Input: dimensioned drawing with shaded views. Units: mm. Origin: part minimum x, y, z. A direction names the side the tool comes from. Give positions to 0.01 mm unless a question says otherwise; leave off trailing zeros. Write each loop counter-clockwise with the first axis right and the second up, starting at its lowest first coordinate (ties: lowest second). Pieces come first, ordered by that corner, then holes.
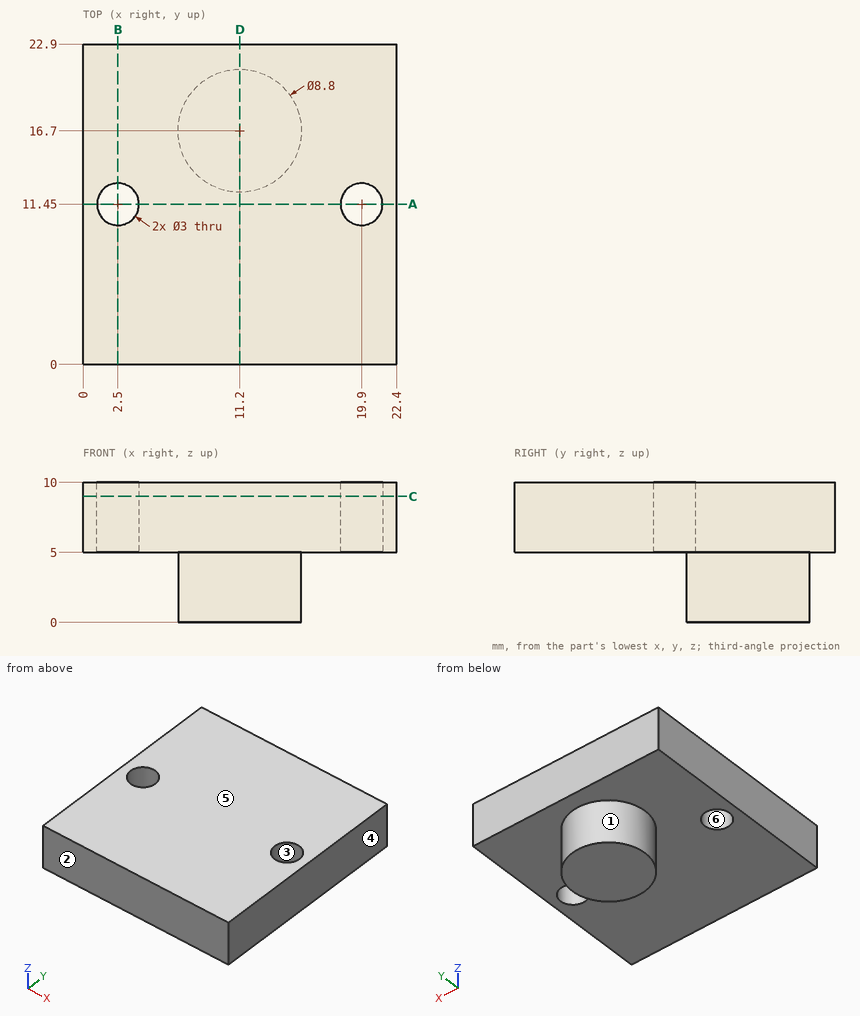
Item 1: Section C-C (z = 9). Return loops of the section in (x, y).
Item 2: Ray query, line 1 (Y direction, x = 19.9, z = 6.7); line 2 (Z direction, x = 1.75, y = 4.25); line 3 (Y direction, x = 11.5, z = 2.25). Return the intervals inside material, ascending.
Item 3: Set-up query: the marked faces 1 and 2. Return all of +Z, -Z, +X, -X, +Y, -Y with unobstructed straight access to the full face (end or side cutting, diameter ignored); none if empty.
Item 4: Section D-D (x = 11.2). Return loops of the section in (y, z).
Item 5: Mould query, pull axis X, two halves, no side actions, for the marked faces 3, 4, 5 and 6. Classes: +X half, -X half, draft (parallel to the pull), parting line (faces both ways), or undercut.
Item 6: Section B-B (x = 2.5). Return loops of the section in (y, z), and give its area (3 significant figures).
Item 7: Section A-A (y = 11.45). Return loops of the section in (x, z), and give its area (3 significant figures).
Item 8: Pin query (flat end, axial travel): pin 1 (1 mm diameter, centred on y = 15.5, z = 4, fed in from -X); pin 2 (5 mm diameter, centred on x = 19.9, y = 11.45, fed in from -Z). Return the tip coordinate at first contact, or that it passes through.
Solved:
1. outline: (0, 0) - (22.4, 0) - (22.4, 22.9) - (0, 22.9) - close; hole circle Ø3 at (2.5, 11.45); hole circle Ø3 at (19.9, 11.45)
2. line 1: y = 0 to 9.95, 12.95 to 22.9
2. line 2: z = 5 to 10
2. line 3: y = 12.31 to 21.09
3. face 1: -Z
3. face 2: +Z, -Z, +X, -X, -Y
4. outline: (0, 5) - (12.3, 5) - (12.3, 0) - (21.1, 0) - (21.1, 5) - (22.9, 5) - (22.9, 10) - (0, 10) - close
5. face 3: undercut
5. face 4: +X half
5. face 5: draft
5. face 6: undercut
6. outline: (0, 5) - (9.95, 5) - (9.95, 10) - (0, 10) - close; (12.95, 5) - (22.9, 5) - (22.9, 10) - (12.95, 10) - close
6. area: 99.5 mm2
7. outline: (0, 5) - (1, 5) - (1, 10) - (0, 10) - close; (4, 5) - (18.4, 5) - (18.4, 10) - (4, 10) - close; (21.4, 5) - (22.4, 5) - (22.4, 10) - (21.4, 10) - close
7. area: 82.0 mm2
8. pin 1: stops at x = 6.86
8. pin 2: stops at z = 5
